Geometry: final body of the model. Coordinates: model frame, mm. Face numbers are marked on the shaded views. A direction names the side the tool comes from. Round coordinates to 2 decimals unless told otherwise and drop trailing zeros. Loops run counter-clockwise (first coordinate to the right, second up) from the corner with the lowest first, then second, coordinate; pieces in that order, holes last. Notation, with made-up numbers: M -3.5,-13.75 L 47.5,-13.75 A27 ccw 47.5,22.25 Z; hole C 81.25,-2 d5. An arc over 180 degrees is marked long. Return JSON: item names as keys, results as strings.
Autodesk Fusion 360 part; units mm, degrees
sketch "Plate" plane through (0, 0, 0) normal (0, 1, 0) x (1, 0, 0)
  line L0 (0, 0) -> (11, 0)
  line L1 (11, 0) -> (11, -48)
  line L2 (11, -48) -> (0, -48)
  line L3 (0, -48) -> (0, 0)
  dimension "d382" = 11
  dimension "d383" = 48
extrude "Plate (1)" add sketch "Plate" along normal mid plane 33 from surface at 4.5
sketch "Hook profile" plane through (0, 0, 0) normal (0, 1, 0) x (1, 0, 0)
  line L0 (0, -46) -> (-8.3, -46)
  line L1 (-8.3, -46) -> (-8.3, -29)
  line L2 (-8.3, -29) -> (-5.3, -29)
  line L3 (-5.3, -29) -> (-3.8, -30.5)
  line L4 (-3.8, -30.5) -> (-3.8, -41)
  line L5 (-3.8, -41) -> (0, -41)
  line L6 (0, -41) -> (0, -46)
  dimension "d387" = 46
  dimension "d388" = 8.3
  dimension "d389" = 3.8
  dimension "d390" = 5
  dimension "d391" = 10.5
  dimension "d392" = 1.5
  dimension "d393" = 1.5
extrude "Hook profile (1)" add sketch "Hook profile" along normal mid plane 2.4
pattern_linear "Hook rows" count 2 spacing 25.4 along (0, 0, -1) count 3 spacing 0 along (0, 0, 1) of "Hook profile (1)"
sketch "Screw hole" plane through (0, 0, 0) normal (0, 1, 0) x (1, 0, 0)
  line L0 (-1, -21.6) -> (12, -21.6)
  line L1 (12, -21.6) -> (12, -26.4)
  line L2 (12, -26.4) -> (-1, -26.4)
  line L3 (-1, -26.4) -> (-1, -21.6)
  dimension "d400" = 12
  dimension "d401" = 21.6
  dimension "d402" = 13
  dimension "d403" = 4.8
extrude "Screw hole (1)" cut sketch "Screw hole" along normal mid plane 16.8 from surface at 7.52
sketch "Nut cavity" plane through (0, 0, 0) normal (0, 1, 0) x (1, 0, 0)
  line L0 (3.6, -20.3) -> (7, -20.3)
  line L1 (7, -20.3) -> (7, -27.7)
  line L2 (7, -27.7) -> (3.6, -27.7)
  line L3 (3.6, -27.7) -> (3.6, -20.3)
  dimension "d407" = 7
  dimension "d408" = 20.3
  dimension "d409" = 3.4
  dimension "d410" = 7.4
extrude "Nut cavity (1)" cut sketch "Nut cavity" along normal mid plane 19.4 from surface at 7.52
sketch "Nut entry" plane through (0, 0, 0) normal (0, 1, 0) x (1, 0, 0)
  line L0 (3.6, -26.7) -> (7, -26.7)
  line L1 (7, -26.7) -> (7, -49)
  line L2 (7, -49) -> (3.6, -49)
  line L3 (3.6, -49) -> (3.6, -26.7)
  dimension "d414" = 7
  dimension "d415" = 26.7
  dimension "d416" = 3.4
  dimension "d417" = 22.3
extrude "Nut entry (1)" cut sketch "Nut entry" along normal mid plane 7.4 from surface at 1.52
sketch "Cavity roof" plane through (0, 0, 0) normal (0, 0, 1) x (1, 0, 0)
  line L0 (3.6, -2.18) -> (7, -2.18)
  line L1 (7, -2.18) -> (5.3, -3.88)
  line L2 (5.3, -3.88) -> (3.6, -2.18)
  dimension "d421" = 3.6
  dimension "d422" = 2.18
  dimension "d423" = 7
  dimension "d424" = 5.3
  dimension "d425" = 1.7
extrude "Cavity roof (1)" cut sketch "Cavity roof" along normal mid plane 29.7 from surface at 34.15
equation "bracketWidth = 24.0 mm"
equation "plateHeight = 48.0 mm"
equation "plateInboardExtension = 9.0 mm"
equation "boardThickness = 6.0 mm"
equation "screwLength = 15.0 mm"
equation "screwDiameter = 4.0 mm"
equation "screwClearance = 0.8 mm"
equation "screwTipClearance = 2.0 mm"
equation "screwSlotWidth = screwDiameter + screwClearance"
equation "nutAcrossFlats = 7.0 mm"
equation "nutThickness = 3.0 mm"
equation "nutChannelClearance = 0.4 mm"
equation "nutChannelHeight = nutAcrossFlats + nutChannelClearance"
equation "plateThickness = screwLength - boardThickness + screwTipClearance"
equation "mountTravel = 12.0 mm"
equation "nutChannelLength = mountTravel + nutAcrossFlats + nutChannelClearance"
equation "screwSlotLength = mountTravel + screwSlotWidth"
equation "topMountZ = 24.0 mm"
equation "mountOffsetY = 7.52 mm"
equation "slotOvershoot = 1.0 mm"
equation "slotWidth = 3.2 mm"
equation "slotPitchVertical = 25.4 mm"
equation "faceMetalThickness = 2.0 mm"
equation "hookTabWidth = slotWidth - 0.8 mm"
equation "hookThroat = faceMetalThickness + 1.8 mm"
equation "hookNeckHeight = 5.0 mm"
equation "hookLipThickness = 4.5 mm"
equation "hookLipDrop = 12.0 mm"
equation "hookLipChamfer = 1.5 mm"
equation "topHookNeckTop = plateHeight - 2 mm"
equation "nutCavityClearance = 0.4 mm"
equation "nutWallThickness = 4.0 mm"
equation "nutCavityDepth = nutThickness + nutCavityClearance"
equation "nutRoofDepth = nutCavityDepth / 2"
equation "d382 = plateThickness"
equation "d383 = plateHeight"
equation "d384 = plateInboardExtension / 2"
equation "d385 = bracketWidth + plateInboardExtension"
equation "d387 = topHookNeckTop"
equation "d388 = hookThroat + hookLipThickness"
equation "d389 = hookThroat"
equation "d390 = hookNeckHeight"
equation "d391 = hookLipDrop - hookLipChamfer"
equation "d392 = hookLipChamfer"
equation "d393 = hookLipChamfer"
equation "d394 = hookTabWidth"
equation "d400 = plateThickness + slotOvershoot"
equation "d401 = topMountZ - screwSlotWidth / 2"
equation "d402 = plateThickness + 2 * slotOvershoot"
equation "d403 = screwSlotWidth"
equation "d404 = mountOffsetY"
equation "d405 = screwSlotLength"
equation "d407 = plateThickness - nutWallThickness"
equation "d408 = topMountZ - nutChannelHeight / 2"
equation "d409 = nutCavityDepth"
equation "d410 = nutChannelHeight"
equation "d411 = mountOffsetY"
equation "d412 = nutChannelLength"
equation "d414 = plateThickness - nutWallThickness"
equation "d415 = topMountZ + nutChannelHeight / 2 - slotOvershoot"
equation "d416 = nutCavityDepth"
equation "d417 = plateHeight - topMountZ - nutChannelHeight / 2 + 2 * slotOvershoot"
equation "d418 = mountOffsetY - mountTravel / 2"
equation "d419 = nutChannelHeight"
equation "d421 = plateThickness - nutWallThickness - nutCavityDepth"
equation "d422 = -( mountOffsetY - nutChannelLength / 2 )"
equation "d423 = plateThickness - nutWallThickness"
equation "d424 = plateThickness - nutWallThickness - nutCavityDepth / 2"
equation "d425 = nutRoofDepth"
equation "d426 = ( topMountZ - nutChannelHeight / 2 + plateHeight ) / 2"
equation "d427 = plateHeight - topMountZ + nutChannelHeight / 2 + 2 * slotOvershoot"
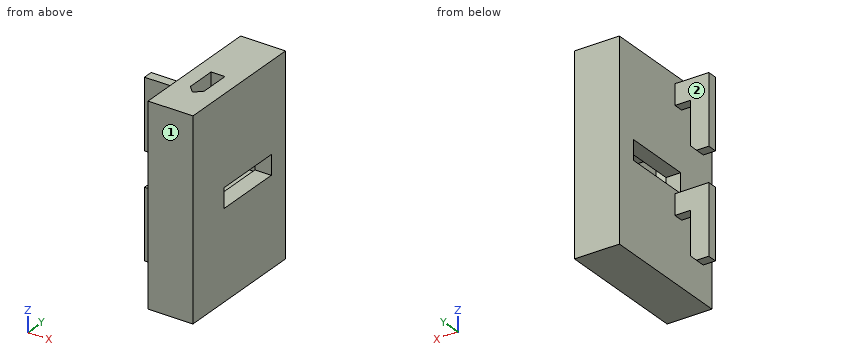
Q1. Section query D-D (z = 11). Output: boundary loops of the cut face in (x, y).
Determined:
{"outline": "M -8.3,-1.2 L -3.8,-1.2 L -3.8,1.2 L -8.3,1.2 Z; M 0,-12 L 11,-12 L 11,21 L 0,21 Z"}
Q2. Pin query (flat end, axial travel): pin 1 (2.5 mm diameter, centred on x = -4, y = 0.5, fed in from +Z); pin 2 (1 mm diameter, centred on x = -4.5, z = 42.5, fed in from +Y); pin 3 (1 mm diameter, centred on y = 9.5, z = 35, fed in from -X); pin 4 (4 mm diameter, centred on x = -2.5, y = 14.5, fed in from -Z). Return the tip coordinate at first contact, or that it passes through.
Determined:
{"pin 1": "stops at z = 46", "pin 2": "stops at y = 1.2", "pin 3": "stops at x = 0", "pin 4": "passes through"}
Q3. Section query B-B (y = 15). Output: boundary loops of the cut face in (x, z), plus the area to 3 significant figures.
Determined:
{"outline": "M 0,0 L 11,0 L 11,21.6 L 7,21.6 L 7,20.3 L 3.6,20.3 L 3.6,21.6 L 0,21.6 Z; M 0,26.4 L 3.6,26.4 L 3.6,27.7 L 7,27.7 L 7,26.4 L 11,26.4 L 11,48 L 0,48 Z", "area": "466 mm^2"}
Q4. Reachability of the marked faces 1 and 2 from +Z, -Z, +X, -X, +Y, -Y: full face, straight path, thin tool, end or side. Return the list, or none.
Determined:
{"face 1": "+Z, -Z, +X, -X, -Y", "face 2": "+Z, -Z, -X, +Y"}
Q5. Section query A-A (z = 36). Output: boundary loops of the cut face in (x, y), plus the area to 3 significant figures.
Determined:
{"outline": "M -8.3,-1.2 L -3.8,-1.2 L -3.8,1.2 L -8.3,1.2 Z; M 0,-12 L 11,-12 L 11,21 L 0,21 Z; hole M 3.6,-2.18 L 5.3,-3.88 L 7,-2.18 L 7,5.22 L 3.6,5.22 Z", "area": "346 mm^2"}
Q6. Material intervals for L1, parallel to X at y = 16, z = 24; L2, parallel to Z at x = 2.75, y = 9; L3, parallel to Y at x = 3.5, z = 25, sorted ascending.
Determined:
{"L1": "x = 0 to 3.6, 7 to 11", "L2": "z = 0 to 21.6, 26.4 to 48", "L3": "y = -12 to -0.88, 15.92 to 21"}
Q7. Section query C-C (x = 10). Output: boundary loops of the cut face in (y, z), plus the area to 3 significant figures.
Determined:
{"outline": "M -12,0 L 21,0 L 21,48 L -12,48 Z; hole M -0.88,21.6 L 15.92,21.6 L 15.92,26.4 L -0.88,26.4 Z", "area": "1,500 mm^2"}
